For this review, use the dimensioned drawing (mm, ordinates from the lowest corner) and the shaded views. A direction names the side the tool comes from. Give positions to 0.01 mm unless a question says otherwise; leave off trailing zeros. Write each loop counter-clockwise with the first axis right and the second up, starting at its lowest first coordinate (ties: lowest second). Pieces come first, ordered by that corner, then holes. Notation, with made-up numbers: M -38,21 L 7,21 A19 ccw 7,42 Z; hole C 31,-29 d7. An arc over 180 degrees is marked long. One line per item, written item: value. Start each with the question number.
Item 1: Consider section A-A, the plane z = 18.5. Write out the cut boundary in (x, y).
Item 2: Tool access review of the marked faces 4 and 5: name each direction out of +Z, -Z, +X, -X, +Y, -Y from which nothing blocks a thin tool from reaching the whole face with its end or side.
Item 3: Consider section B-B, the plane x = 93. Write out the cut boundary in (y, z), and give its area (3 significant figures).
Item 4: Clearance check with flat-ended pins moving along their axes: pin 1 Ø1.5 at (y, z) = (52, 17.5) entering from -X; pin 2 Ø4 at (x, y) = (36, 109.5) entering from +Z. State where each tip first meets the part, or that it passes through.
Item 5: Mouldability with a two-part tool opening along X and no side actions: class the marked faces 1, 2 and 3 as released by +X, released by -X, zero draft, split by the parting line, or undercut.
Item 6: To check wall thickness, follow probe 1 along Y at (x, z) = (49, 18.5); probe 2 along Z at (x, y) = (94.5, 68). State the ranges of each line that lie inside material, in increasing order.
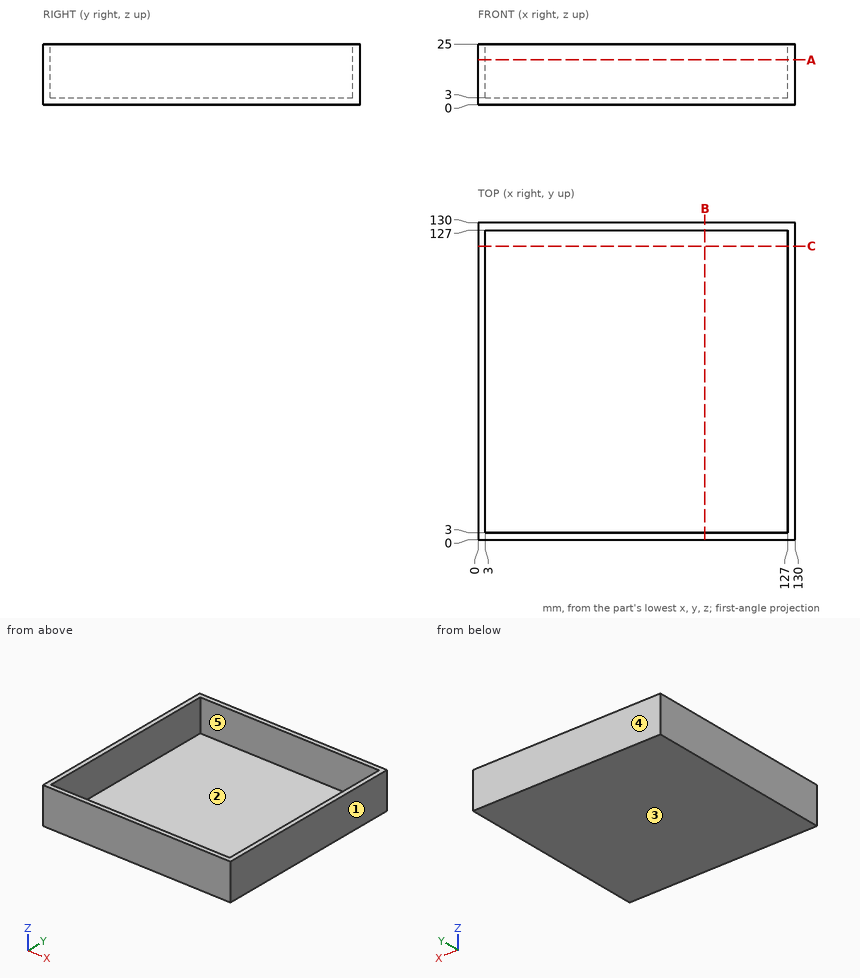
Model answer:
1. outline: M 0,0 L 130,0 L 130,130 L 0,130 Z; hole M 3,3 L 127,3 L 127,127 L 3,127 Z
2. face 4: +Z, -Z, +X, -X, +Y
2. face 5: +Z
3. outline: M 0,0 L 130,0 L 130,25 L 127,25 L 127,3 L 3,3 L 3,25 L 0,25 Z
3. area: 522 mm2
4. pin 1: stops at x = 0
4. pin 2: stops at z = 3
5. face 1: released by +X
5. face 2: undercut
5. face 3: zero draft
6. probe 1: y = 0 to 3, 127 to 130
6. probe 2: z = 0 to 3
